```python
from build123d import *

# Parameters (mm, degrees)
ARM_DEPTH               = 6.35
CUT_EXTRUDE1_DEPTH      = 100.058228154
CUT_EXTRUDE1_DEPTH_BACK = 100.058228154
SKETCH2_R               = 1.27
CUT_EXTRUDE2_DEPTH      = 100.058228154
CUT_EXTRUDE2_DEPTH_BACK = 100.058228154
SKETCH3_R               = 1.27
FILLET2_R               = 6.35
FILLET3_R               = 2.54
CHAMFER1_SIZE           = 3.81


with BuildPart() as part:
    # Sketch1 → Arm (new body)
    with BuildSketch(Plane(origin=(0, 0, 0), x_dir=(1, 0, 0), z_dir=(0, 1, 0))):
        Polygon((0, -19.058070864), (97, -13.588070864), (97, -8.5), (84.3, -9.216175258), (84.3, 9.216175258), (97, 8.5), (97, 13.588070864), (0, 19.058070864), (0, 13.97), (12.7, 13.253824742), (12.7, -13.253824742), (0, -13.97), align=None)
        Polygon((79.22, -9.502645361), (51.04, -11.091764948), (51.04, 11.091764948), (79.22, 9.502645361), align=None, mode=Mode.SUBTRACT)
        Polygon((17.78, 12.967354639), (17.78, -12.967354639), (45.96, -11.378235052), (45.96, 11.378235052), align=None, mode=Mode.SUBTRACT)
    extrude(amount=ARM_DEPTH)

    # Sketch2 → Cut-Extrude1 (cut, two sides: drawn at the far end of the back side and taken through both)
    with BuildSketch(Plane.XY.offset(-CUT_EXTRUDE1_DEPTH_BACK)):
        with Locations(Location((30.48, 3.175, 0), (0, 0, 180))):
            Circle(SKETCH2_R)
    extrude(amount=CUT_EXTRUDE1_DEPTH + CUT_EXTRUDE1_DEPTH_BACK, mode=Mode.SUBTRACT)

    # Sketch3 → Cut-Extrude2 (cut, two sides: drawn at the far end of the back side and taken through both)
    with BuildSketch(Plane.XY.offset(-CUT_EXTRUDE2_DEPTH_BACK)):
        with Locations((93.19, 3.175)):
            Circle(SKETCH3_R)
        with Locations(Location((3.81, 3.175, 0), (0, 0, 180))):
            Circle(SKETCH3_R)
    extrude(amount=CUT_EXTRUDE2_DEPTH + CUT_EXTRUDE2_DEPTH_BACK, mode=Mode.SUBTRACT)

    # Fillet2
    fillet2_edges = [part.edges().sort_by_distance(p)[0] for p in [
        (12.7, 3.175, 13.253824742),
        (12.7, 3.175, -13.253824742),
        (84.3, 3.175, -9.216175258),
        (84.3, 3.175, 9.216175258),
        (45.96, 3.175, -11.378235052),
        (17.78, 3.175, -12.967354639),
        (17.78, 3.175, 12.967354639),
        (45.96, 3.175, 11.378235052),
        (79.22, 3.175, 9.502645361),
        (79.22, 3.175, -9.502645361),
        (51.04, 3.175, -11.091764948),
        (51.04, 3.175, 11.091764948),
    ]]
    fillet(fillet2_edges, radius=FILLET2_R)

    # Fillet3
    fillet3_edges = [part.edges().sort_by_distance(p)[0] for p in [
        (97, 6.35, 11.044035432),
        (0, 0, -16.514035432),
        (97, 0, -11.044035432),
        (97, 0, 11.044035432),
        (0, 0, 16.514035432),
        (97, 6.35, -11.044035432),
        (0, 6.35, -16.514035432),
        (0, 6.35, 16.514035432),
    ]]
    fillet(fillet3_edges, radius=FILLET3_R)

    # Chamfer1
    # the kernel refuses this chamfer: 3.81 mm, written as the material it takes off along each edge
    with BuildSketch(Plane(origin=(17.78, 6.35, -6.24917843), x_dir=(0.027495876610586382, -0.9996219169112968, 0), z_dir=(0, 0, 1))) as chamfer1_piece_1:
        Polygon((CHAMFER1_SIZE * 0.999621916911, -CHAMFER1_SIZE * 0.0274958766106), (-CHAMFER1_SIZE * 0.0274958766106, -CHAMFER1_SIZE * 0.999621916911), (0, 0), align=None)
    extrude(amount=12.49835686, mode=Mode.SUBTRACT)
    with BuildSketch(Plane(origin=(24.13, 6.35, 6.24917843), x_dir=(0.9995733988743083, 0, -0.02920651062456478), z_dir=(-0.02920651062456478, 0, -0.9995733988743083))) as chamfer1_piece_2:
        Polygon((6.35, CHAMFER1_SIZE), (6.35 + CHAMFER1_SIZE, 0), (6.35, 0), align=None)
    revolve(axis=Axis((24.13, 6.35, 6.24917843), (0, -1, 0)), revolution_arc=181.673647793, mode=Mode.SUBTRACT)
    with BuildSketch(Plane(origin=(24.13, 6.35, -6.24917843), x_dir=(0.9995733988743084, 0, 0.029206510624563663), z_dir=(-0.029206510624563663, 0, 0.9995733988743084))) as chamfer1_piece_3:
        Polygon((6.35, -CHAMFER1_SIZE), (6.35 + CHAMFER1_SIZE, 0), (6.35, 0), align=None)
    revolve(axis=Axis((24.13, 6.35, -6.24917843), (0, 1, 0)), revolution_arc=181.673647793, mode=Mode.SUBTRACT)


solid = part.part
```
Model file for the job. Use its own axes, mm. A direction names the side the tool comes from. Coordinates: 2 decimals unless noted, no trailing zeros. Order: outer loops, then holes, each group sorted by start corner. A loop starts at its lowest first (then second) coordinate and runs counter-clockwise, first axis right, second up. Notation, with made-up numbers: (77.5, -7) -> (101.5, -7) arc R9 ccw to (101.5, 0) -> close; hole circle Ø4 at (-2, -30). An arc over 180 degrees is marked (long way). Answer as a JSON object with one key per item and string values. Group by question number.
1) Drill centre lines: L1, parallel to Y at x = 93.19, z = 11.05 (3 decimals); L2, parallel to X at y = 5, z = -1; L3, parallel to X at y = 4, z = -1.5. Where is each one in solid material? Low to high.
2) Cut at A-A, the plane x = 93.19. Write the cut outline in (y, z) (3 decimals), then the cut area to 3 significant figures.
3) Pull direction Y, two halves, no side cores. Call faces 1 (the face through (96.236, 0.724, 11.079)), 2 (the face through (3.22, 4.3, 16.26)), 3 (the face through (47.82, 3.13, 16.36)): +Y half, -Y half, draft (parallel to the pull), parting line (faces both ways), or undercut.
4) Cut at D-D, the plane x = 80.5. Write the cut outline in (y, z).
5) Cut at B-B, the plane x = 36. Write the cut outline in (y, z).
6) Flat gauge pins, fed straight in: pin 1 (1.5 mm diameter, centred on y = 4.5, z = 0.5, fed in from +X); pin 2 (3 mm diameter, centred on x = 47.5, y = 2, fed in from +Z); pin 3 (1.9 mm diameter, centred on y = 4.5, z = -1, fed in from -X). Where does each tip first touch, or does it go through?
7) Cut at C-C, the plane z = 15. Count the separate pieces of the cut face and the enclosed holes in it, then the cut area to 3 significant figures.
8) Which spindle directions (+Z, -Z, +X, -X, +Y, -Y) get a long thin tool onto all of the face, cutting with end or side? Do faces 4 (the face through (10.92, 3.22, 11.66)), 5 (the face through (34.06, 2.42, -12.05)), 6 (the face through (0.724, 5.586, -16.406)). Say none if no direction does.
Check values:
{
 "1": {"L1": "y = 0 to 1.905, 4.445 to 6.35", "L2": "x = 12.7 to 15.32, 45.96 to 51.04, 79.22 to 84.3", "L3": "x = 12.7 to 16.32, 45.96 to 51.04, 79.22 to 84.3"},
 "2": {"outline": "(0, -13.803) -> (1.905, -13.803) -> (1.905, -8.715) -> (0, -8.715) -> close; (0, 8.715) -> (1.905, 8.715) -> (1.905, 13.803) -> (0, 13.803) -> close; (4.445, -13.803) -> (6.35, -13.803) -> (6.35, -8.715) -> (4.445, -8.715) -> close; (4.445, 8.715) -> (6.35, 8.715) -> (6.35, 13.803) -> (4.445, 13.803) -> close", "area": "38.8 mm²"},
 "3": {"face 1": "-Y half", "face 2": "undercut", "face 3": "draft"},
 "4": {"outline": "(0, -14.52) -> (6.35, -14.52) -> (6.35, 14.52) -> (0, 14.52) -> close"},
 "5": {"outline": "(0, -17.03) -> (6.35, -17.03) -> (6.35, -11.94) -> (0, -11.94) -> close; (0, 11.94) -> (6.35, 11.94) -> (6.35, 17.03) -> (0, 17.03) -> close"},
 "6": {"pin 1": "stops at x = 84.3", "pin 2": "stops at z = 16.46", "pin 3": "stops at x = 12.7"},
 "7": {"separate pieces": "1", "enclosed holes": "2", "area": "435 mm²"},
 "8": {"face 4": "-X, +Y, -Y", "face 5": "+Y, -Y", "face 6": "+Z, -Z, -X, +Y"}
}
